For this review, use the dimensioned drawing (mm, ordinates from the lowest corner) and the shaded views. A direction names the side the tool comes from. Round coordinates to 2 decimals unless told otherwise and drop trailing zeros. Write each loop counter-clockwise with the first axis right and the second up, starting at its lowest first coordinate (ties: lowest second). Pieces come first, ordered by that corner, then holes.
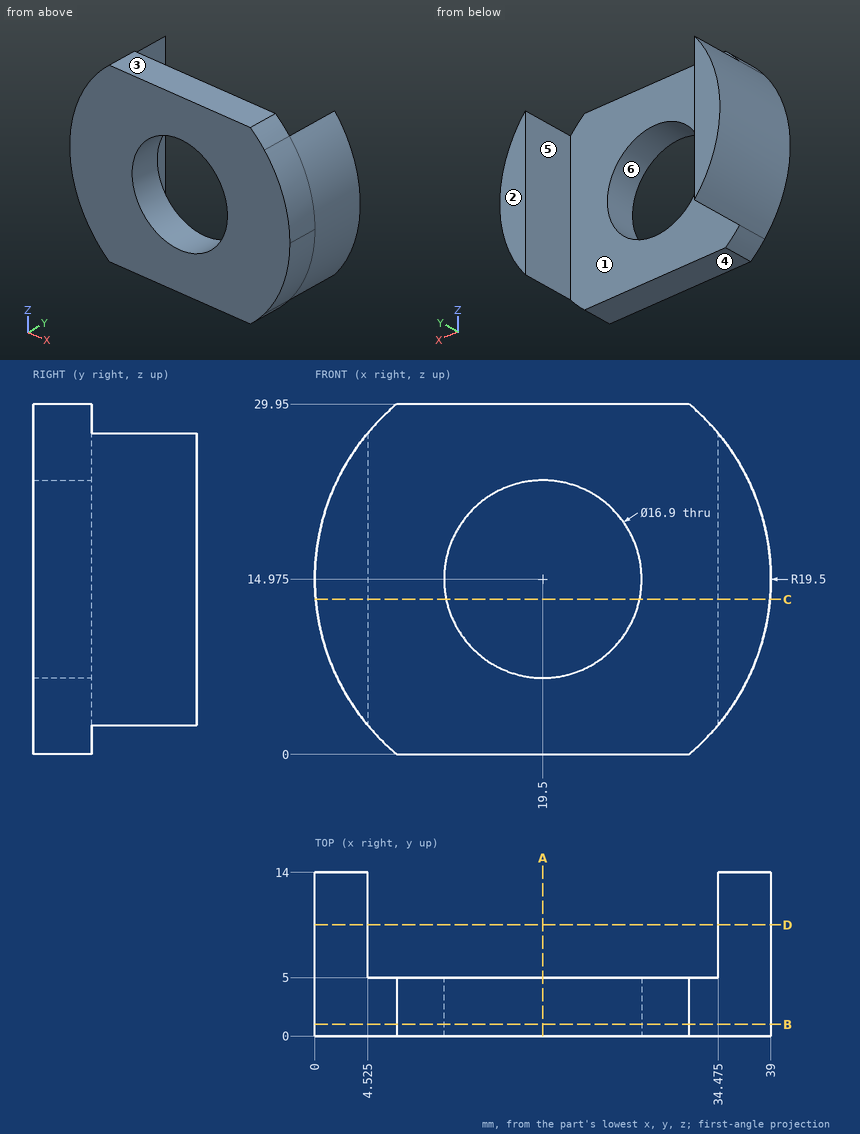
1) For line 1 along Z through (x, y) = (19.5, 2.55) (3 decimals); line 2 along X through (y, z) = (11, 14.5) (3 decimals); line 3 along Y through (x, z) = (18, 27.5), list the stretches that pass through material, from the lowest coordinate up.
2) Add section D-D on y = 9.5. State the section outline as (x, z) points (3 decimals), and give its area (3 significant figures).
3) For P1, Ø5, axis at y = 8.5, z = 10, coming from the +X side; P2, Ø15, axis at x = 19.5, z = 14.975, coming from the -Y side; P3, Ø5, axis at y = 6.5, z = 3.5, coming from the +X side; P4, Ø1, axis at y = 11.5, z = 23.5, coming from the -X side, all flat-tipped, find the tip position at first contact; note any pin that passes through.
4) Add section C-C on z = 13.25. State the section outline as (x, y) points (3 decimals), and give its area (3 significant figures).
5) Add section A-A on x = 19.5. State the section outline as (y, z) points (3 decimals).
6) Add section B-B on y = 1. State the section outline as (x, z) points (3 decimals), and give its area (3 significant figures).
7) The part is to be moulded in two halves that separate along Z. For the marked faces 3, 4, 5 and 6, say which applies: pulls with the +Z half, pulls with the -Z half, needs draft (parallel to the pull), parting line crosses it, or undercut.
8) For the marked faces 1 and 2, list the 3-axis set-ups (+Z, -Z, +X, -X, +Y, -Y) from which the entire face can be reached by the end or side of a thin tool; tool diameter is ignored.
Computed:
1. line 1: z = 0 to 6.525, 23.425 to 29.95
1. line 2: x = 0.006 to 4.525, 34.475 to 38.994
1. line 3: y = 0 to 5
2. outline: (4.525, 2.485) - (4.525, 27.465) arc R19.5 ccw to start; (34.475, 2.485) arc R19.5 ccw to (34.475, 27.465) - close
2. area: 155 mm2
3. P1: stops at x = 38.84
3. P2: passes through
3. P3: stops at x = 36.81
3. P4: stops at x = 1.73
4. outline: (0.076, 0) - (11.228, 0) - (11.228, 5) - (4.525, 5) - (4.525, 14) - (0.076, 14) - close; (27.772, 0) - (38.924, 0) - (38.924, 14) - (34.475, 14) - (34.475, 5) - (27.772, 5) - close
4. area: 192 mm2
5. outline: (0, 0) - (5, 0) - (5, 6.525) - (0, 6.525) - close; (0, 23.425) - (5, 23.425) - (5, 29.95) - (0, 29.95) - close
6. outline: (7.01, 0) - (31.99, 0) arc R19.5 ccw to (31.99, 29.95) - (7.01, 29.95) arc R19.5 ccw to start; hole circle Ø16.9 at (19.5, 14.975)
6. area: 816 mm2
7. face 3: pulls with the +Z half
7. face 4: pulls with the -Z half
7. face 5: needs draft
7. face 6: undercut
8. face 1: +Z, -Z, +Y
8. face 2: +Z, -Z, +X, -X, +Y
